Can you work these out from the drawing? Everything is in mm from the part's minimum corner. A direction names the side the tool comes from. Give positions to 0.01 mm unless a question says otherwise; leave off trailing zeros. Loops run counter-clockwise (first coordinate to the right, second up) from the corner with the lowest first, then second, coordinate; pieces in that order, holes last. Notation, with made-up numbers: (27, 21.5) - (73, 21.5) arc R10 cw to (73, 37.5) - close; hole circle Ø1 at (-36.75, 30). An arc over 180 degrees is marked (long way). One line per item, written item: value. Start each with the question number.
Q1. I'm going to push flat-ended pins straight in: P1, Ø1.2, axis at y = 37, z = 2.5, coming from the -X side; P2, Ø4, axis at y = 11, z = 15.5, coming from the +X side; P3, Ø11, axis at x = 21, y = 16, coming from the +Z side. Where does each tip first touch, or does it pass through?
Q2. I want a section at A-A (z = 74.6). Please give me the cut outline in (x, y).
Q3. I want a section at D-D (z = 110.5). Please give me the cut outline in (x, y) (1 decimal), then the cut area to 3 significant figures.
Q4. I want a section at C-C (y = 4.5). Please give me the cut outline in (x, z), then the cut area to 3 significant figures.
Q5. If I drill on line 1 (X direction, y = 36.25, z = 74.6); line 2 (Y direction, x = 65.5, z = 103); line 3 (Z direction, x = 34.5, y = 13.5), over which ranges is the centre line in solid material (lowest first)? Write a range as from..to.
Q6. I want a section at B-B (x = 84). Please give me the cut outline in (y, z) (1 decimal), then the cut area to 3 significant figures.
Q7. For the marked faces 4, 5 and 6, which set-ups out of +Z, -Z, +X, -X, +Y, -Y let a thin tool reach every point of the face, with its end or its side?
Q8. If we mould it in two halves opening along X, with no side actions, what happens to the marked faces 1, 2 and 3? For each: released by +X, released by -X, zero draft, split by the parting line, or undercut.
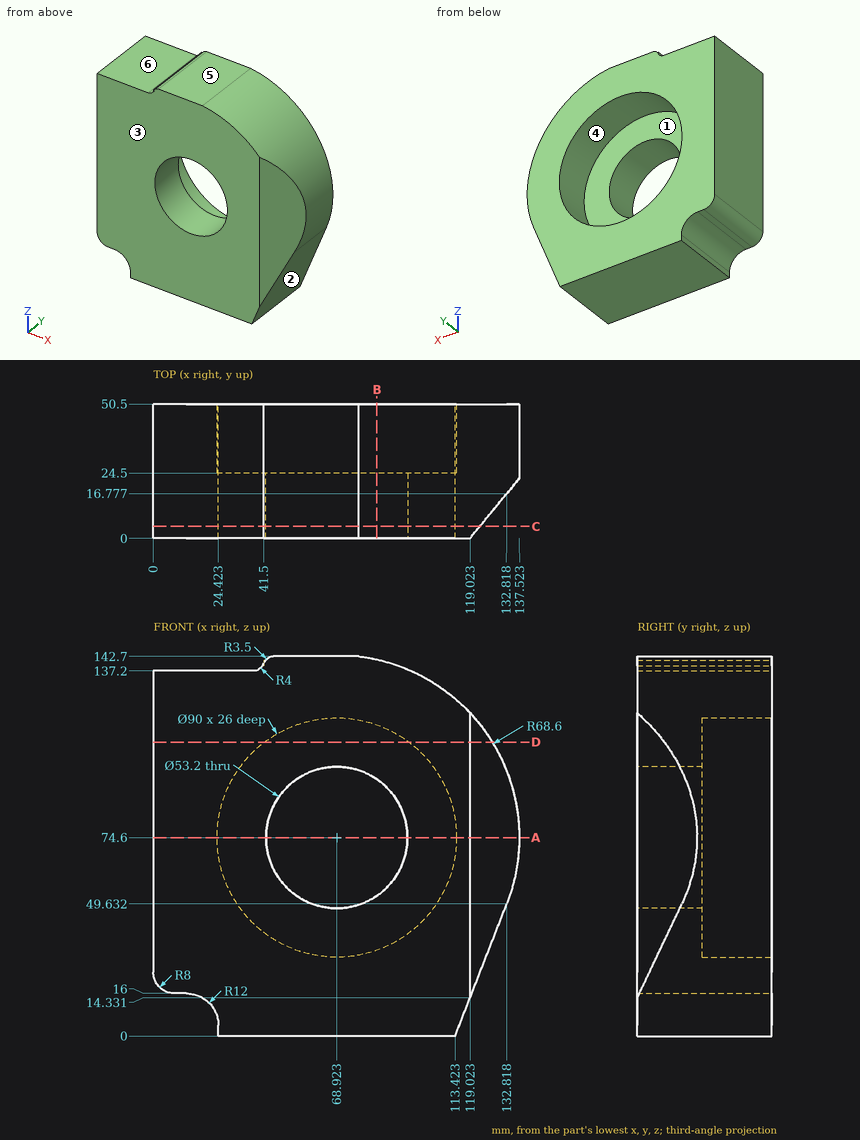
Worked answers:
1. P1: stops at x = 24.42
1. P2: stops at x = 120.26
1. P3: stops at z = 137.2
2. outline: (0, 0) - (42.32, 0) - (42.32, 24.5) - (23.92, 24.5) - (23.92, 50.5) - (0, 50.5) - close; (95.52, 0) - (119.02, 0) - (137.52, 22.5) - (137.52, 50.5) - (113.92, 50.5) - (113.92, 24.5) - (95.52, 24.5) - close
3. outline: (0, 0) - (119, 0) - (127.4, 10.2) - (127.4, 50.5) - (96.1, 50.5) - (96.1, 24.5) - (41.8, 24.5) - (41.8, 50.5) - (0, 50.5) - close
3. area: 4,980 mm²
4. outline: (0, 24) arc R8 ccw to (8, 16) - (12.42, 16) arc R12 cw to (24.42, 4) - (24.42, 0) - (113.42, 0) - (122.72, 23.8) - (122.72, 117.16) arc R68.6 ccw to (77.19, 142.7) - (45, 142.7) arc R3.5 ccw to (41.5, 139.2) - (41.5, 141.2) arc R4 cw to (37.5, 137.2) - (0, 137.2) - close; hole circle Ø53.2 at (68.92, 74.6)
4. area: 14,200 mm²
5. line 1: x = 0..23.92, 113.92..137.52
5. line 2: y = 0..24.5
5. line 3: z = 0..137.2
6. outline: (0, 0) - (50.5, 0) - (50.5, 32.2) - (24.5, 32.2) - (24.5, 52.7) - (0, 52.7) - close; (0, 96.5) - (24.5, 96.5) - (24.5, 117) - (50.5, 117) - (50.5, 141.5) - (0, 141.5) - close
6. area: 3,870 mm²
7. face 4: +Y
7. face 5: +Z, +X, -X, +Y, -Y
7. face 6: +Z, -X, +Y, -Y
8. face 1: undercut
8. face 2: released by +X
8. face 3: zero draft
